Read the model definition and answer for the solid it produces. Units are mm, in the model's axes. A direction names the side the tool comes from. Coordinates: 2 decimals unless noted, no trailing zeros. Loops run counter-clockwise (first coordinate to the right, second up) from the corner with the lowest first, then second, coordinate; pieces in that order, holes last. Notation, with made-up numbers: (75.25, 58) -> (117.25, 58) arc R25 cw to (117.25, 74) -> close; hole circle Ø2 at (32.5, 42). An arc over 180 degrees is marked (long way). Answer as CSV lines item,"result".
Autodesk Inventor part; units mm, degrees
ref_plane "YZ Plane" through (0, 0, 0) normal (1, 0, 0) x (0, 1, 0)
ref_plane "XZ Plane" through (0, 0, 0) normal (0, 1, 0) x (-1, 0, 0)
ref_plane "XY Plane" through (0, 0, 0) normal (0, 0, 1) x (1, 0, 0)
sketch "スケッチ1" plane through (0, 0, 0) normal (0, 0, 1) x (1, 0, 0)
  line L0 (-10, -20) -> (10, -20)
  line L1 (10, -20) -> (10, 20)
  line L2 (10, 20) -> (-10, 20)
  line L3 (-10, 20) -> (-10, -20)
  line L4 (-10, -20) -> (10, 20) construction
  line L5 (10, -20) -> (-10, 20) construction
  point P0 (0, 0)
  dimension "d0" = 20
  dimension "d1" = 40
extrude "押し出し1" add sketch "スケッチ1" along normal blind 25
sketch "スケッチ2" plane through (10, -20, 0) normal (1, 0, 0) x (0, 0, -1)
  circle A0 centre (-25, 20) radius 11.1
  line L0 (0, 40) -> (-25, 40)
  dimension "d4" = 22.2
  dimension "d7" = 20
extrude "押し出し2" cut sketch "スケッチ2" against normal through all
sketch "スケッチ7" plane through (0, 0, 0) normal (1, 0, 0) x (0, 1, 0)
  arc A0 (-11.1, 25) -> (11.1, 25) centre (0, 25) ccw
  line L0 (20, 25) -> (11.1, 25)
  line L1 (20, 0) -> (20, 25)
  line L2 (20, 0) -> (-20, 0)
  line L3 (-20, 0) -> (-20, 25)
  line L4 (-11.1, 25) -> (-20, 25)
  circle A1 centre (0, 25) radius 6
  arc A2 (-11.1, 25) -> (11.1, 25) centre (0, 25) ccw
  line L5 (11.1, 25) -> (-11.1, 25)
  point P0 (0, 0)
  point P1 (-6, 25)
  point P2 (6, 25)
  dimension "d27" = 12
extrude "押し出し5" add sketch "スケッチ7" along normal mid plane 10 contours L5 A1 A0
sketch "スケッチ5" plane through (0, 0, 25) normal (0, 0, 1) x (1, 0, 0)
  line L0 (10, 20) -> (-10, 20)
  line L1 (-10, -20) -> (10, -20)
  point P0 (0, 0)
  point P1 (0, 10)
  point P2 (0, -10)
  dimension "d18" = 10
  dimension "d19" = 10
hole "穴1" at (0, 10, 25) at (0, -10, 25) direction (0, 0, -1) diameter 5.3 depth 58
sketch "Sketch9" plane through (-10, -20, 0) normal (-1, 0, 0) x (0, 0, 1)
  arc A0 (25, 31.1) -> (25, 8.9) centre (25, 20) ccw
  line L0 (25, 40) -> (25, 31.1)
  line L1 (0, 40) -> (25, 40)
  line L2 (0, 40) -> (0, 0)
  line L3 (0, 0) -> (25, 0)
  line L4 (25, 8.9) -> (25, 0)
  point P0 (0, 20)
extrude "Extrusion7" add sketch "Sketch9" along normal blind 18
sketch "Sketch10" plane through (0, 0, 0) normal (0, 0, -1) x (-1, 0, 0)
  circle A0 centre (0, 10) radius 2.65
  circle A1 centre (0, -10) radius 2.65
  line L0 (28, -20) -> (-10, -20)
  line L1 (28, 20) -> (28, -20)
  line L2 (-10, 20) -> (28, 20)
  line L3 (-10, -20) -> (-10, 20)
  line L4 (-10, -20) -> (-10, -11.1)
  line L5 (-10, 20) -> (28, 20)
  line L6 (-10, -20) -> (10, -20)
  line L7 (10, -20) -> (10, 20)
  line L8 (10, 20) -> (-10, 20)
  line L9 (-10, 20) -> (-10, -20)
  point P0 (0, 0)
  dimension "d34" = 20
extrude "Extrusion8" add sketch "Sketch10" along normal blind 20 contours L0 L7 L2 L1
sketch "Sketch11" plane through (-5, 0, 0) normal (-1, 0, 0) x (0, 0, 1)
  line L0 (0, 7.35) -> (25, 7.35)
  line L1 (25, -11.1) -> (25, -6)
  arc A0 (25, 6) -> (25, -6) centre (25, 0) ccw
  line L2 (25, 6) -> (25, 11.1)
  arc A1 (25, 11.1) -> (25, -11.1) centre (25, 0) ccw
  point P0 (0, 0)
extrude "Extrusion9" add sketch "Sketch11" along normal blind 18
chamfer "Chamfer2" distance 10 angle 45 1 edges at (-28, 0, -20)
sketch "Sketch12" plane through (0, 0, 25) normal (0, 0, 1) x (1, 0, 0)
  line L0 (10, -20) -> (10, -11.1)
  circle A0 centre (0, -10) radius 2.65
  line L1 (10, -11.1) -> (5, -11.1)
  line L2 (5, -6) -> (5, -11.1)
  line L3 (5, -6) -> (-23, -6)
  line L4 (-23, -11.1) -> (-23, -6)
  line L5 (-23, -11.1) -> (-28, -11.1)
  line L6 (-28, -20) -> (-28, -11.1)
  line L7 (10, -20) -> (-28, -20)
  line L8 (10, -20) -> (10, -11.1)
  circle A1 centre (0, 10) radius 2.65
  line L9 (-28, 11.1) -> (-23, 11.1)
  line L10 (-23, 6) -> (-23, 11.1)
  line L11 (-23, 6) -> (5, 6)
  line L12 (5, 11.1) -> (5, 6)
  line L13 (5, 11.1) -> (10, 11.1)
  line L14 (10, 11.1) -> (10, 20)
  line L15 (10, 20) -> (-28, 20)
  line L16 (-28, 11.1) -> (-28, 20)
  point P0 (0, 0)
  point P1 (-18, -10)
  point P2 (-18, 10)
  dimension "d42" = 28
hole "Hole2" at (-18, -10, 25) at (-18, 10, 25) direction (0, 0, -1) diameter 5.4 depth 10
chamfer "Chamfer3" distance 2 angle 45 8 edges at (10, -20, 12.5) (10, 20, 12.5) (-28, -20, 7.5) (-28, 20, 7.5) (-23, 20, -15) (-23, -20, -15) (-14, 20, -20) (-14, -20, -20)
sketch "スケッチ13" plane through (-28, -20, 0) normal (-1, 0, 0) x (0, 0, 1)
  line L0 (-20, 38) -> (-10, 38)
  line L1 (-20, 38) -> (-20, 2)
  line L2 (-10, 2) -> (-20, 2)
  line L3 (-10, 2) -> (-10, 38)
  line L4 (-9.1716, 0) -> (25, 0)
  line L5 (25, 0) -> (25, 2)
  line L6 (25, 2) -> (-10, 2)
  line L7 (-9.1716, 0) -> (-10, 2)
  line L8 (-10, 38) -> (25, 38)
  line L9 (25, 38) -> (25, 40)
  line L10 (25, 40) -> (-9.1716, 40)
  line L11 (-9.1716, 40) -> (-10, 38)
  point P0 (0, 20)
  point P1 (-10, 10)
  point P2 (-10, 30)
  dimension "d53" = 10
  dimension "d54" = 10
hole "穴3" at (-28, -10, -10) at (-28, 10, -10) direction (1, 0, 0) diameter 4.3 end through all counterbore diameter 8 counterbore depth 13
sketch "スケッチ14" plane through (-15, -10, -10) normal (-1, 0, 0) x (0, 0, 1)
  circle A0 centre (0, 0) radius 2.15
  circle A1 centre (0, 20) radius 4
  circle A2 centre (0, 20) radius 2.15
  line L0 (2.15, -2.15) -> (-2.15, -2.15)
  line L1 (-2.15, -2.15) -> (-2.15, 2.15)
  line L2 (-2.15, 2.15) -> (2.15, 2.15)
  line L3 (2.15, 2.15) -> (2.15, -2.15)
  line L4 (2.15, -2.15) -> (-2.15, 2.15) construction
  line L5 (-2.15, -2.15) -> (2.15, 2.15) construction
  line L6 (2.15, 17.85) -> (-2.15, 17.85)
  line L7 (-2.15, 17.85) -> (-2.15, 22.15)
  line L8 (-2.15, 22.15) -> (2.15, 22.15)
  line L9 (2.15, 22.15) -> (2.15, 17.85)
  line L10 (2.15, 17.85) -> (-2.15, 22.15) construction
  line L11 (-2.15, 17.85) -> (2.15, 22.15) construction
  circle A3 centre (0, 20) radius 2.15
  point P0 (10, 10)
extrude "押し出し10" cut sketch "スケッチ14" against normal blind 0.6 contours A0 | L3 L0 A0 | A0 L2 L3 | A0 L1 L2 | L0 L1 A0 | A2 | L9 L6 A2 | A2 L8 L9 | A2 L7 L8 | L6 L7 A2
sketch "スケッチ15" plane through (-15, -10, -10) normal (-1, 0, 0) x (0, 0, 1)
  line L0 (2.15, -2.15) -> (-2.15, -2.15)
  line L1 (-2.15, 2.15) -> (2.15, 2.15)
  circle A0 centre (0, 0) radius 4
  line L2 (-2.15, -16.7131) -> (2.15, -16.7131)
  line L3 (2.15, -16.7131) -> (2.15, 35.0465)
  line L4 (2.15, 35.0465) -> (-2.15, 35.0465)
  line L5 (-2.15, 35.0465) -> (-2.15, -16.7131)
  line L6 (-2.15, 17.85) -> (-2.15, 22.15)
  line L7 (-2.15, 22.15) -> (2.15, 22.15)
  line L8 (2.15, 22.15) -> (2.15, 17.85)
  line L9 (2.15, 17.85) -> (-2.15, 17.85)
  circle A1 centre (0, 20) radius 4
  point P0 (10, 10)
  point P1 (-2.15, -3.3731)
  point P2 (2.15, -3.3731)
  point P3 (-2.15, 3.3731)
  point P4 (2.15, 3.3731)
  point P5 (2.15, 23.3731)
  point P6 (-2.15, 23.3731)
  point P7 (-2.15, 16.6269)
  point P8 (2.15, 16.6269)
extrude "押し出し11" cut sketch "スケッチ15" against normal blind 0.3 contours L3 A0 L5 L0 | L1 L5 A0 L3 | A1 L5 L9 L3 | A1 L3 L7 L5
properties part number "Print_Parts_L" material "PC/ABS プラスチック"
Q1. Find the intervals of material crossed by probe 1 along Y at (x, z) = (-20.75, -10); probe 2 along Y at (x, z) = (-11.3, -10); probe 3 along Z at (x, y) = (-13, -10), in increasing order. Write a range as [from, to].
Results:
probe 1,"y = [-20, -14], [-6, 6], [14, 20]"
probe 2,"y = [-20, -12.15], [-7.85, 7.85], [12.15, 20]"
probe 3,"z = [-20, -12.15], [-7.85, 25]"
Q2. Given pin 1 Ø1.1 at (y, z) = (-8.5, -11.5) entering from -X; pin 2 Ø5 at (y, z) = (-6.5, -10.5) entering from +X; pin 3 Ø0.6 at (y, z) = (11, -13) entering from -X, each flat-ended and moving along its own axis, determine where each tip first touches the part or whether it passes through.
Results:
pin 1,"stops at x = -14.4"
pin 2,"stops at x = -10"
pin 3,"stops at x = -15"
Q3. For a pull along X with two mould halves and no side action, classify faces 5 (the face through (10, 0, 10)), 6 (the face through (-0.117, -7.353, 12.325)), 7 (the face through (-9, 0, 19)) as pulls with the +X half, pulls with the -X half, needs draft (parallel to the pull), parting line crosses it, or undercut.
Results:
face 5,"pulls with the +X half"
face 6,"undercut"
face 7,"needs draft"
Q4. A cutting plane is placed at D-D, the plane y = -15.5. Write down the section's boundary in (x, z).
Results:
outline,"(-28, -10) -> (-18, -20) -> (-10, -20) -> (-10, 0) -> (10, 0) -> (10, 25) -> (-28, 25) -> close"
Q5. A cutting plane is placed at C-C, the plane x = -20. Write down the section's boundary in (y, z), and give its area (3 significant figures).
Results:
outline,"(-20, -15.17) -> (-18, -18) -> (18, -18) -> (20, -15.17) -> (20, 25) -> (11.81, 25) -> (11.81, 15) -> (8.19, 15) -> (8.19, 25) -> (6, 25) arc R6 cw to (-6, 25) -> (-8.19, 25) -> (-8.19, 15) -> (-11.81, 15) -> (-11.81, 25) -> (-20, 25) -> close; hole circle Ø8 at (-10, -10); hole circle Ø8 at (10, -10)"
area,"1,480 mm²"
Q6. For faces 1 (the face through (-20.677, 10.351, 19.93)), 2 (the face through (7.5, -0.2, 13.9)), 3 (the face through (-14.4, -8, -8)), 4 (the face through (-10, 0, -10)), determine the directions among +Z, -Z, +X, -X, +Y, -Y from which every point of the face is accessible in a straight line to the end or side of a thin tool.
Results:
face 1,"+Z"
face 2,"+Z, +X"
face 3,"-X"
face 4,"-Z, +X, +Y, -Y"
Q7. A cutting plane is placed at A-A, the plane x = 0. Write down the section's boundary in (y, z), and give its area (3 significant figures).
Results:
outline,"(-20, 0) -> (-12.65, 0) -> (-12.65, 25) -> (-20, 25) -> close; (-7.35, 0) -> (7.35, 0) -> (7.35, 25) -> (6, 25) arc R6 cw to (-6, 25) -> (-7.35, 25) -> close; (12.65, 0) -> (20, 0) -> (20, 25) -> (12.65, 25) -> close"
area,"678 mm²"
Q8. A cutting plane is placed at B-B, the plane y = 0. Write down the section's boundary in (x, z).
Results:
outline,"(-28, -10) -> (-18, -20) -> (-10, -20) -> (-10, 0) -> (10, 0) -> (10, 13.9) -> (5, 13.9) -> (5, 19) -> (-23, 19) -> (-23, 13.9) -> (-28, 13.9) -> close"
